Part model, mm, in its own coordinate system. Face numbers are marked on the shaded views. A direction names the side the tool comes from. Coordinates: 2 decimals unless noted, no trailing zeros. Loops run counter-clockwise (first coordinate to the right, second up) from the corner with the lowest first, then second, coordinate; pieces in that order, holes last. Notation, with made-up numbers: (-36.75, 55.25) - (5.25, 55.25) arc R20 cw to (5.25, 87.25) - close; hole circle Ø11 at (35, -27). An arc over 180 degrees is marked (long way). One line per question, with ' | ' between items. Start each with the question number.
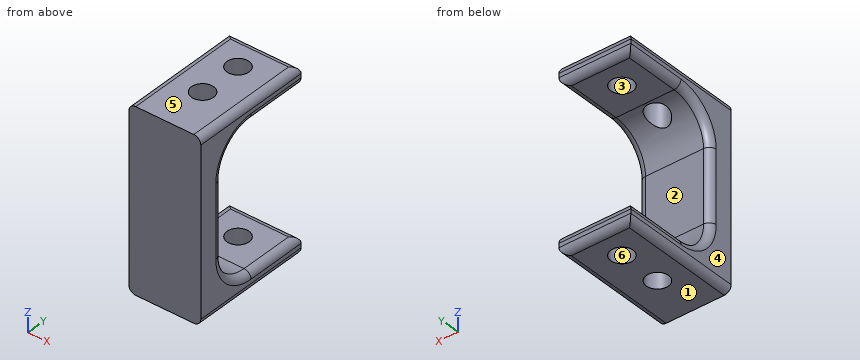
from build123d import *

# Parameters (mm, degrees)
F1_DEPTH     = 10
F2_R         = 1.538196108
F3_DEPTH     = 25
F4_T4_DEPTH  = 10
F4_S5_R      = 1.538196108
F4_T6_DEPTH  = 8
F4_T10_DEPTH = 10
F4_S11_R     = 1.538196108
F4_T12_DEPTH = 8
F5_R         = 0.9656854249


# Not quite as in the source:
# - a fillet or chamfer that OpenCascade refuses, or shapes differently, is made with other operations: its cross-section is extruded or revolved along the edge and cut away or added


with BuildPart() as f1:
    # F0 (on Right) → F1 (new body)
    with BuildSketch(Plane.YZ):
        Polygon((17, 0), (0, 0), (0, -25), (17, -25), (17, -22.5), (3.5, -22.5), (3.5, -2.5), (17, -2.5), align=None)
    extrude(amount=F1_DEPTH)

    # F2 (on face) → F3 (cut)
    with BuildSketch(Plane(origin=(0, 0, -25), x_dir=(1, 0, 0), z_dir=(0, 0, -1))):
        with Locations((4.8035508953, -6.6337394528)):
            Circle(F2_R)
        with Locations((4.8077256637, -12.6337380004)):
            Circle(F2_R)
    extrude(amount=-F3_DEPTH, mode=Mode.SUBTRACT)

    # F4: fillet of radius 5 on 2 edges, made by hand


with BuildPart() as f4_tool2:
    # F4_s3 → F4_t4 (new body)
    with BuildSketch(Plane.YZ):
        with BuildLine():
            ThreePointArc((8.5, -2.5), (4.9644660941, -3.9644660941), (3.5, -7.5))
            Line((3.5, -7.5), (3.5, -2.5))
            Line((3.5, -2.5), (8.5, -2.5))
        make_face()
    extrude(amount=F4_T4_DEPTH)

    # F4_s5 → F4_t6 (cut, symmetric)
    with BuildSketch(Plane.XY.offset(-5)):
        with Locations((4.8035508953, 6.6337394528)):
            Circle(F4_S5_R)
    extrude(amount=F4_T6_DEPTH, both=True, mode=Mode.SUBTRACT)


with BuildPart() as f1_1:
    add(f1.part)

    # F4_t1: union F4_tool2
    add(f4_tool2.part)


with BuildPart() as f4_tool8:
    # F4_s9 → F4_t10 (new body)
    with BuildSketch(Plane.YZ):
        with BuildLine():
            ThreePointArc((8.5, -22.5), (4.9644660941, -21.0355339059), (3.5, -17.5))
            Line((3.5, -17.5), (3.5, -22.5))
            Line((3.5, -22.5), (8.5, -22.5))
        make_face()
    extrude(amount=F4_T10_DEPTH)

    # F4_s11 → F4_t12 (cut, symmetric)
    with BuildSketch(Plane.XY.offset(-20)):
        with Locations((4.8035508953, 6.6337394528)):
            Circle(F4_S11_R)
    extrude(amount=F4_T12_DEPTH, both=True, mode=Mode.SUBTRACT)


with BuildPart() as f1_2:
    add(f1_1.part)

    # F4_t7: union F4_tool8
    add(f4_tool8.part)

    # F5
    f5_edges = [f1_2.edges().sort_by_distance(p)[0] for p in [
        (5, 17, -22.5),
        (5, 17, -25),
        (5, 17, 0),
        (5, 17, -2.5),
        (0, 8.5, 0),
        (10, 8.5, 0),
        (10, 8.5, -25),
        (0, 8.5, -25),
        (10, 4.964466, -3.964466),
        (0, 4.964466, -3.964466),
        (0, 3.5, -12.5),
    ]]
    fillet(f5_edges, radius=F5_R)


solid = f1_2.part
1) Tool access for the marked faces 1 and 2: list every direction of +Z, -Z, +X, -X, +Y, -Y with a clear straight run to the whole face (end or side of a thin tool).
2) Band-saw the part on D-D on x = 2.25. List the corners of the cut face in (y, z).
3) Band-saw the part on B-B on x = 4.5. Count the separate pieces of the cut face and the enclosed holes in it, then the cut area to 3 significant figures.
4) Pin check, flat tips, straight feed: pin 1 Ø1.8 at (x, y) = (4.81, 12.63) entering from -Z; pin 2 Ø2.5 at (x, z) = (6, -14.5) entering from +Y. Stop position of each tip, or through.
5) Mould opens along X. For the marked faces 3, 4, 5 and 6 say: +X half, -X half, draft (parallel to the pull), parting line (faces both ways), or undercut.
6) Band-saw the part on C-C on z = -8.75. List the corners of the cut face in (x, y), then the cut area to 3 significant figures.
7) Wall check: line 1 along Z through (x, y) = (5.75, 8.5); line 2 along Y through (x, z) = (1.75, -9); line 3 along Z through (x, y) = (2, 7.25). Give the ranges that are in metal, low to high. Write a range as [from, to].
8) Band-saw the part on A-A on y = 14.75. List the corners of the cut face in (x, z).
Values found:
1) face 1: -Z, +X, -X, +Y, -Y | face 2: +X, -X, +Y
2) outline: (0, -25) - (16.03, -25) arc R0.97 ccw to (17, -24.03) - (17, -23.47) arc R0.97 ccw to (16.03, -22.5) - (8.5, -22.5) arc R5 cw to (3.5, -17.5) - (3.5, -7.5) arc R5 cw to (8.5, -2.5) - (16.03, -2.5) arc R0.97 ccw to (17, -1.53) - (17, -0.97) arc R0.97 ccw to (16.03, 0) - (0, 0) - close
3) separate pieces: 5 | enclosed holes: 0 | area: 132 mm²
4) pin 1: through | pin 2: y = 3.5
5) face 3: undercut | face 4: -X half | face 5: draft | face 6: undercut
6) outline: (0, 0) - (10, 0) - (10, 2.53) arc R0.97 ccw to (9.03, 3.5) - (0.97, 3.5) arc R0.97 ccw to (0, 2.53) - close | area: 34.6 mm²
7) line 1: [-25, -22.5], [-2.5, 0] | line 2: [0, 3.5] | line 3: [-25, -22.34], [-2.66, 0]
8) outline: (0, -24.03) arc R0.97 ccw to (0.97, -25) - (9.03, -25) arc R0.97 ccw to (10, -24.03) - (10, -23.47) arc R0.97 ccw to (9.03, -22.5) - (0.97, -22.5) arc R0.97 ccw to (0, -23.47) - close; (0, -1.53) arc R0.97 ccw to (0.97, -2.5) - (9.03, -2.5) arc R0.97 ccw to (10, -1.53) - (10, -0.97) arc R0.97 ccw to (9.03, 0) - (0.97, 0) arc R0.97 ccw to (0, -0.97) - close
